Work out the finished part from the listing and answer in its coordinate system (mm). Face numbers are marked on the shaded views. A direction names the side the tool comes from. Round coordinates to 2 decimals unless told otherwise and drop trailing zeros. Order: outer loops, then holes, each group sorted by start corner. A loop starts at its lowest first (then second) coordinate and runs counter-clockwise, first axis right, second up. Notation, with made-up numbers: (70, 49) - (108, 49) arc R18 cw to (108, 58) - close; hole circle Ø3 at (-34.75, 73.5). An arc over 180 degrees is marked (long way). Put each result on its own line as item: value.
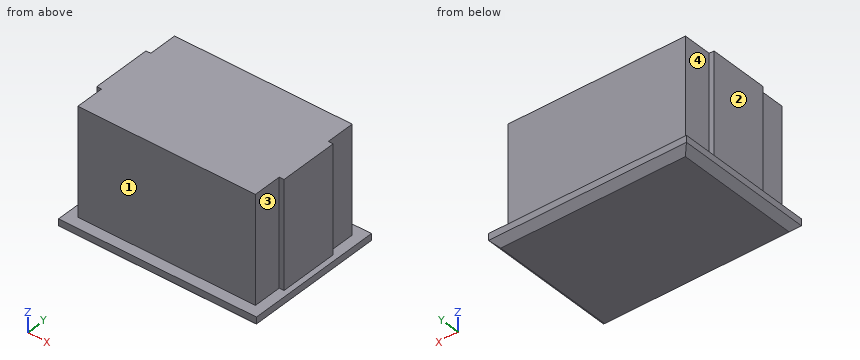
```python
from build123d import *

# Parameters (mm, degrees)
SKETCH1_W           = 13.28
SKETCH1_H           = 8.75
BOSS_EXTRUDE1_DEPTH = 8
SKETCH2_W           = 14.8
SKETCH2_H           = 10.4
BOSS_EXTRUDE2_DEPTH = 1
CHAMFER2_SIZE       = 0.5
SKETCH3_W           = 14
SKETCH3_H           = 4.45
BOSS_EXTRUDE3_DEPTH = 8


with BuildPart() as part:
    # Sketch1 → Boss-Extrude1 (new body)
    with BuildSketch(Plane.XY):
        Rectangle(SKETCH1_W, SKETCH1_H)
    extrude(amount=BOSS_EXTRUDE1_DEPTH)

    # Sketch2 → Boss-Extrude2 (add)
    with BuildSketch(Plane(origin=(0, 0, 0), x_dir=(-1, 0, 0), z_dir=(0, 0, -1))):
        Rectangle(SKETCH2_W, SKETCH2_H)
    extrude(amount=BOSS_EXTRUDE2_DEPTH)

    # Chamfer2
    chamfer2_edges = [part.edges().sort_by_distance(p)[0] for p in [
        (7.4, 0, -1),
        (0, -5.2, -1),
        (-7.4, 0, -1),
        (0, 5.2, -1),
    ]]
    chamfer(chamfer2_edges, length=CHAMFER2_SIZE)

    # Sketch3 → Boss-Extrude3 (add)
    with BuildSketch(Plane.XY.offset(8)):
        Rectangle(SKETCH3_W, SKETCH3_H)
    extrude(amount=-BOSS_EXTRUDE3_DEPTH)


solid = part.part
```
1) A cutting plane is placed at B-B on y = 0. Write down the section's boundary in (x, z), then the cut area to 3 significant figures.
Findings below:
outline: (-7.4, -0.5) - (-6.9, -1) - (6.9, -1) - (7.4, -0.5) - (7.4, 0) - (7, 0) - (7, 8) - (-7, 8) - (-7, 0) - (-7.4, 0) - close
area: 127 mm2
2) Straight lines are drawn through the part: L1, parallel to Z at x = 6.5, y = 4.5; L2, parallel to Y at x = 3.5, z = 1 (3 decimals); L3, parallel to X at y = 2.75, z = 6. For each, find the intervals that lie inside material, in ascending order. Write a range as from..to.
Findings below:
L1: z = -1..0
L2: y = -4.375..4.375
L3: x = -6.64..6.64
3) A cutting plane is placed at C-C on x = 4.5. Write down the section's boundary in (y, z) (3 decimals).
Findings below:
outline: (-5.2, -0.5) - (-4.7, -1) - (4.7, -1) - (5.2, -0.5) - (5.2, 0) - (4.375, 0) - (4.375, 8) - (-4.375, 8) - (-4.375, 0) - (-5.2, 0) - close
4) Given pin 1 Ø4 at (y, z) = (-2, 4) entering from +X; pin 2 Ø1.1 at (y, z) = (3, 2.5) entering from +X; pin 3 Ø4 at (x, z) = (4, 2.5) entering from -Y (3 decimals), each flat-ended and moving along its own axis, determine where each tip first touches the part or whether it passes through.
Findings below:
pin 1: stops at x = 7
pin 2: stops at x = 6.64
pin 3: stops at y = -4.375
5) A cutting plane is placed at A-A on z = 0.25. Write down the section's boundary in (x, y) (3 decimals), then the cut area to 3 significant figures.
Findings below:
outline: (-7, -2.225) - (-6.64, -2.225) - (-6.64, -4.375) - (6.64, -4.375) - (6.64, -2.225) - (7, -2.225) - (7, 2.225) - (6.64, 2.225) - (6.64, 4.375) - (-6.64, 4.375) - (-6.64, 2.225) - (-7, 2.225) - close
area: 119 mm2
6) For the marked faces 1, 2, 3 and 4, determine the directions among +Z, -Z, +X, -X, +Y, -Y from which every point of the face is accessible in a straight line to the end or side of a thin tool.
Findings below:
face 1: +Z, +X, -X, -Y
face 2: +Z, -X, +Y, -Y
face 3: +Z, +X, -Y
face 4: +Z, -X, +Y
